```python
from build123d import *

# Parameters (mm, degrees)
F1_DEPTH = 25.4
F2_W     = 12.7
F2_H     = 12.7
F3_DEPTH = 25.4
F4_W     = 12.7
F4_H     = 12.7
F5_DEPTH = 12.7


with BuildPart() as f1:
    # F0 (on Front) → F1 (new body)
    with BuildSketch(Plane.XZ):
        Polygon((0, 25.4), (0, 0), (38.1, 0), (38.1, 12.7), (6.35, 12.7), (6.35, 25.4), align=None)
    extrude(amount=F1_DEPTH)

    # F2 (on face) → F3 (cut)
    with BuildSketch(Plane.YZ.offset(6.35)):
        with Locations((-12.7, 19.05)):
            Rectangle(F2_W, F2_H)
    extrude(amount=-F3_DEPTH, mode=Mode.SUBTRACT)

    # F4 (on face) → F5 (cut)
    with BuildSketch(Plane.YZ.offset(38.1)):
        with Locations((-12.466443, 6.35)):
            Rectangle(F4_W, F4_H)
    extrude(amount=-F5_DEPTH, mode=Mode.SUBTRACT)


solid = f1.part
```
Check sheet for the modelled part. Datum: model origin and axes. Units: mm. A direction names the side the tool comes from. Round coordinates to 2 decimals unless told otherwise and drop trailing zeros. Order: outer loops, then holes, each group sorted by start corner. A loop starts at its lowest first (then second) coordinate and runs counter-clockwise, first axis right, second up.
1) Scan lines: line 1 (Y direction, x = 33.5, z = 12.25); line 2 (X direction, y = -4.5, z = 21.75); line 3 (Z direction, x = 34, y = -2). Record each from-to range of solid material in increasing order.
2) Tool access check on faces 1 (the flat face through (6.35, -3, 19)), 2 (the flat face through (3, -6.35, 19)), 3 (the flat face through (32, -18.816, 6)), 4 (the flat face through (38.1, -3, 6)). Record the directions out of +Z, -Z, +X, -X, +Y, -Y that give a thin tool (end or side, any length) a straight path to the whole face; none if there is none.
3) Section check D-D (y = -3). Record the boundary of the cut face in (x, z), and give its area (3 significant figures).
4) Section check C-C (z = 2.75). Record the boundary of the cut face in (x, y), and give its area (3 significant figures).
5) Mould release check, pull along Y, two halves, no side actions. Record for faces 5 (the flat face through (15, 0, 7)), 6 (the flat face through (0, -13, 10)), 7 (the flat face through (3, -19.05, 19)): +Y half, -Y half, draft (parallel to the pull), parting line (faces both ways), or undercut.
6) Section check A-A (z = 22.75). Record the boundary of the cut face in (x, y).
7) Go/stop test with flat-tipped pins: pin 1 Ø8 at (x, y) = (12.5, -10) entering from +Z; pin 2 Ø7 at (y, z) = (-3.5, 18) entering from +X; pin 3 Ø1.5 at (x, z) = (31.5, 14) entering from +Y. Record where each tip stops, or that it passes through.
8) Section check B-B (x = 30). Record the boundary of the cut face in (y, z).
Result:
1. line 1: y = -25.4 to -18.82, -6.12 to 0
1. line 2: x = 0 to 6.35
1. line 3: z = 0 to 12.7
2. face 1: +Z, +X, +Y, -Y
2. face 2: +Z, +X, -X
2. face 3: +Z, -Z, +X
2. face 4: +Z, -Z, +X, +Y, -Y
3. outline: (0, 0) - (38.1, 0) - (38.1, 12.7) - (6.35, 12.7) - (6.35, 25.4) - (0, 25.4) - close
3. area: 565 mm2
4. outline: (0, -25.4) - (38.1, -25.4) - (38.1, -18.82) - (25.4, -18.82) - (25.4, -6.12) - (38.1, -6.12) - (38.1, 0) - (0, 0) - close
4. area: 806 mm2
5. face 5: +Y half
5. face 6: draft
5. face 7: undercut
6. outline: (0, -25.4) - (6.35, -25.4) - (6.35, -19.05) - (0, -19.05) - close; (0, -6.35) - (6.35, -6.35) - (6.35, 0) - (0, 0) - close
7. pin 1: stops at z = 12.7
7. pin 2: stops at x = 6.35
7. pin 3: passes through
8. outline: (-25.4, 0) - (-18.82, 0) - (-18.82, 12.7) - (-25.4, 12.7) - close; (-6.12, 0) - (0, 0) - (0, 12.7) - (-6.12, 12.7) - close
